from build123d import *

# Parameters (mm, degrees)
SKETCH1_W               = 35
SKETCH1_H               = 20
BOSS_EXTRUDE1_DEPTH     = 1.5
SKETCH2_R               = 1.6
CUT_M3_HOLE_DEPTH       = 37.431442464
SKETCH3_R               = 6
BOSS_FSR_BOSS_DEPTH     = 1
FILLET1_R               = 10
SKETCH4_R               = 9.5
SKETCH4_R_2             = 8.5
CUT_EXTRUDE_THIN1_DEPTH = 0.2


with BuildPart() as part:
    # Sketch1 → Boss-Extrude1 (new body)
    with BuildSketch(Plane.XY):
        with Locations((17.5, 0)):
            Rectangle(SKETCH1_W, SKETCH1_H)
    extrude(amount=BOSS_EXTRUDE1_DEPTH)

    # Sketch2 → Cut-M3 Hole (cut, through all)
    with BuildSketch(Plane.XY.offset(1.5)):
        with Locations((5, 0)):
            Circle(SKETCH2_R)
    extrude(amount=-CUT_M3_HOLE_DEPTH, mode=Mode.SUBTRACT)

    # Sketch3 → Boss-FSR Boss (add)
    with BuildSketch(Plane.XY.offset(1.5)):
        with Locations((25, 0)):
            Circle(SKETCH3_R)
    extrude(amount=BOSS_FSR_BOSS_DEPTH)

    # Fillet1
    fillet1_edges = [part.edges().sort_by_distance(p)[0] for p in [
        (0, 10, 0.75),
        (35, 10, 0.75),
        (35, -10, 0.75),
        (0, -10, 0.75),
    ]]
    fillet(fillet1_edges, radius=FILLET1_R - 0.0001)  # a hair under: the kernel refuses the full size

    # Sketch4 → Cut-Extrude-Thin1 (cut)
    with BuildSketch(Plane.XY.offset(1.5)):
        with Locations((25, 0)):
            Circle(SKETCH4_R)
        with Locations((25, 0)):
            Circle(SKETCH4_R_2, mode=Mode.SUBTRACT)
    extrude(amount=-CUT_EXTRUDE_THIN1_DEPTH, mode=Mode.SUBTRACT)


solid = part.part
The model under review builds one solid part; all positions refer to its coordinate system, in mm. A direction names the side the tool comes from. Coordinates: 2 decimals unless noted, no trailing zeros. Write each loop counter-clockwise with the first axis right and the second up, starting at its lowest first coordinate (ties: lowest second). Pieces come first, ordered by that corner, then holes. Notation, with made-up numbers: (50.25, -30) - (59.25, -30) arc R26 cw to (59.25, -12) - close; hole circle Ø8 at (-12, -19.5). An arc over 180 degrees is marked (long way). Answer as CSV lines item,"result".
(1) We need section A-A (x = 5). Give the boundary of the cut face in (y, z).
Data:
outline,"(-8.66, 0) - (-1.6, 0) - (-1.6, 1.5) - (-8.66, 1.5) - close; (1.6, 0) - (8.66, 0) - (8.66, 1.5) - (1.6, 1.5) - close"
(2) Mouldability with a two-part tool opening along Y and no side actions: class faces 3 (the cylindrical face through (2.85, -6.99, 0.76)), 4 (the cylindrical face through (20.24, -3.65, 1.99)), 5 (the cylindrical face through (3.4, 0.07, 0.76)), 6 (the cylindrical face through (2.85, 6.99, 0.76)) as pulls with the +Y half, pulls with the -Y half, needs draft (parallel to the pull), parting line crosses it, or undercut.
Data:
face 3,"pulls with the -Y half"
face 4,"parting line crosses it"
face 5,"undercut"
face 6,"pulls with the +Y half"
(3) Tool access review of faces 1 (the flat face through (25, 0, 2.5)), 2 (the flat face through (22.8, -8.4, 1.3)): name each direction out of +Z, -Z, +X, -X, +Y, -Y from which nothing blocks a thin tool from reaching the whole face with its end or side.
Data:
face 1,"+Z, +X, -X, +Y, -Y"
face 2,"+Z"
(4) We need section D-D (x = 26). Give the boundary of the cut face in (y, z).
Data:
outline,"(-9.95, 0) - (9.95, 0) - (9.95, 1.5) - (9.45, 1.5) - (9.45, 1.3) - (8.44, 1.3) - (8.44, 1.5) - (5.92, 1.5) - (5.92, 2.5) - (-5.92, 2.5) - (-5.92, 1.5) - (-8.44, 1.5) - (-8.44, 1.3) - (-9.45, 1.3) - (-9.45, 1.5) - (-9.95, 1.5) - close"
(5) We need section C-C (y = -7). Give the boundary of the cut face in (x, z).
Data:
outline,"(2.86, 0) - (32.14, 0) - (32.14, 1.5) - (31.42, 1.5) - (31.42, 1.3) - (29.82, 1.3) - (29.82, 1.5) - (20.18, 1.5) - (20.18, 1.3) - (18.58, 1.3) - (18.58, 1.5) - (2.86, 1.5) - close"
(6) For line 1 along Y through (x, z) = (25, 1.4); line 2 along X through (y, z) = (-0.25, 1.35); line 3 along Z through (x, y) = (2, 4), list the stretches that pass through material, from the lowest coordinate up. Write a range as [from, to].
Data:
line 1,"y = [-10, -9.5], [-8.5, 8.5], [9.5, 10]"
line 2,"x = [0, 3.42], [6.58, 15.5], [16.5, 33.5], [34.5, 35]"
line 3,"z = [0, 1.5]"
(7) Clearance check with flat-ended pins moving along their axes: pin 1 Ø3 at (x, y) = (5, 0) entering from -Z; pin 2 Ø4 at (x, y) = (5.5, -2) entering from +Z; pin 3 Ø1.5 at (y, z) = (3.5, 0.5) entering from +X. State where each tip first meets the part, or that it passes through.
Data:
pin 1,"passes through"
pin 2,"stops at z = 1.5"
pin 3,"stops at x = 34.61"
